Verification items for the finished model (mm, model axes). Face numbers are marked on the shaded views. Round coordinates to 2 decimals unless told otherwise and drop trailing zeros. Write each loop counter-clockwise with the first axis right and the second up, starting at its lowest first coordinate (ties: lowest second). Pieces come first, ordered by that corner, then holes. Notation, with made-up numbers: (73, 38.5) - (102, 38.5) arc R16 cw to (102, 69.5) - close; hole circle Ø4 at (58, 42.5). An arc over 180 degrees is marked (long way). Answer as a JSON object with one key per item and string values. Group by question number.
1) Section check C-C (z = 4.25). Enter the section's corners in (x, y), then the cut area to 3 significant figures.
2) Go/stop test with a flat-tipped pin: pin 1 Ø4 at (x, y) = (6, 13) entering from -Z. Record where the tip stops, or that it passes through.
3) Section check A-A (y = 7.5). Enter the section's corners in (x, z).
4) Thickness scan on line 1 (X direction, y = 7.5, z = 5); line 2 (X direction, y = 12, z = 8.75); line 3 (Y direction, x = 9.5, z = 3.5). Record the ranges inside material, lowest first.
5) Section check B-B (x = 11). Enter the section's corners in (y, z).
6) Mould release check, pull along Y, two halves, no side actions. Record for the marked faces 1, 2 and 3: +Y half, -Y half, draft (parallel to the pull), parting line (faces both ways), or undercut.
Autodesk Inventor part; units mm, degrees
ref_plane "YZ Plane" through (0, 0, 0) normal (1, 0, 0) x (0, 1, 0)
ref_plane "XZ Plane" through (0, 0, 0) normal (0, 1, 0) x (-1, 0, 0)
ref_plane "XY Plane" through (0, 0, 0) normal (0, 0, 1) x (1, 0, 0)
sketch "Sketch1" plane through (0, 0, 0) normal (0, 0, 1) x (1, 0, 0)
  point P0 (0, 0)
sketch "Sketch2" plane through (0, 0, 0) normal (0, 0, 1) x (1, 0, 0)
  line L0 (0, 0) -> (15, 0)
  line L1 (15, 0) -> (15, 15)
  line L2 (15, 15) -> (0, 15)
  line L3 (0, 15) -> (0, 0)
  line L4 (0, 7.9375) -> (15.875, 7.9375)
  line L5 (7.9375, 15) -> (7.9375, 0)
  dimension "d0" = 15
  dimension "d1" = 15
extrude "Extrusion1" add sketch "Sketch2" along normal blind 10
sketch "Sketch3" plane through (0, 0, 10) normal (0, 0, 1) x (1, 0, 0)
  line L0 (0, 14.9966) -> (7.5, 15)
  line L1 (15, 15) -> (0, 15)
  line L2 (0.0034, 7.4661) -> (15, 7.2509)
  arc A0 (7.5017, 0) -> (7.5, 15) centre (-22407.2052, 4.9864) ccw
  circle A1 centre (7.5021, 7.5) radius 5.5
  point P0 (0, 0)
  dimension "d4" = 11
extrude "Extrusion2" cut sketch "Sketch3" along normal through all both and the other way through all
thread "Thread1"
properties part number "bolt1"
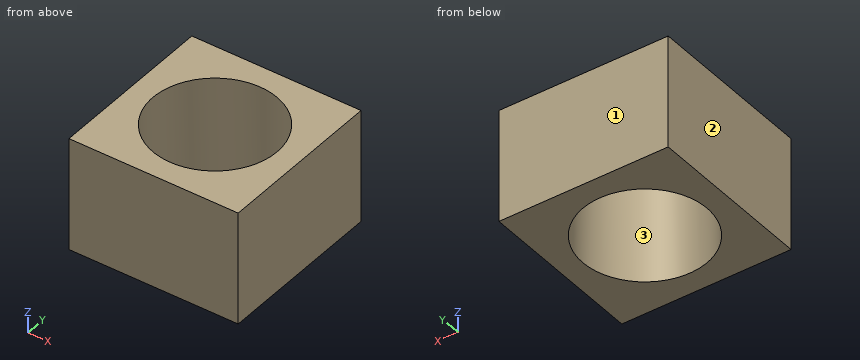
Returned:
{
 "1": {"outline": "(0, 0) - (15, 0) - (15, 15) - (0, 15) - close; hole circle Ø11 at (7.5, 7.5)", "area": "130 mm2"},
 "2": {"pin 1": "z = 0"},
 "3": {"outline": "(0, 0) - (2, 0) - (2, 10) - (0, 10) - close; (13, 0) - (15, 0) - (15, 10) - (13, 10) - close"},
 "4": {"line 1": "0 to 2, 13 to 15", "line 2": "0 to 4.34, 10.66 to 15", "line 3": "0 to 2.38, 12.62 to 15"},
 "5": {"outline": "(0, 0) - (3.26, 0) - (3.26, 10) - (0, 10) - close; (11.74, 0) - (15, 0) - (15, 10) - (11.74, 10) - close"},
 "6": {"face 1": "+Y half", "face 2": "draft", "face 3": "undercut"}
}
